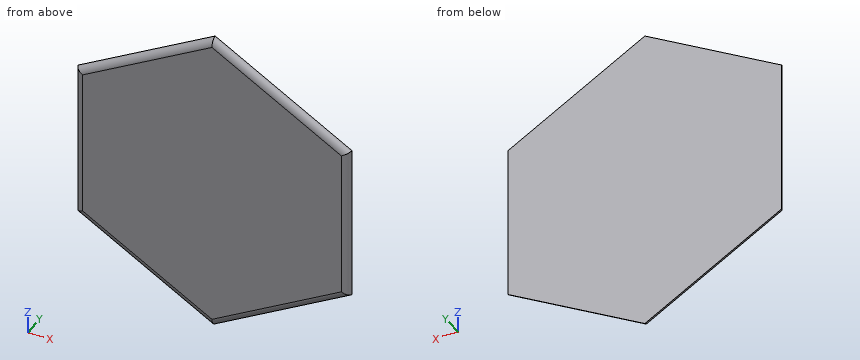
from build123d import *

# Parameters (mm, degrees)
F1_DEPTH     = 4
F2_T1_DEPTH  = 128.417945882
F2_T3_DEPTH  = 128.417945882
F2_T5_DEPTH  = 128.417945882
F2_T7_DEPTH  = 128.417945882
F2_T9_DEPTH  = 128.417945882
F2_T11_DEPTH = 128.417945882


# Not quite as in the source:
# - a fillet or chamfer that OpenCascade refuses, or shapes differently, is made with other operations: its cross-section is extruded or revolved along the edge and cut away or added


with BuildPart() as f1:
    # F0 (on Front) → F1 (new body)
    with BuildSketch(Plane.XZ):
        Polygon((89.9928545723, 51.9738985062), (-0.0142891539, 103.9230474718), (-90.0071437262, 51.9491489656), (-89.9928545723, -51.9738985062), (0.0142891539, -103.9230474718), (90.0071437262, -51.9491489656), align=None)
    extrude(amount=F1_DEPTH)

    # F2: fillet of radius 5 on 6 edges, made by hand

    # F2_s2 → F2_t1 (cut)
    with BuildSketch(Plane(origin=(-0.0088285699, 0, 64.208972334), x_dir=(0, 1, 0), z_dir=(0.0001374974, 0, -0.9999999905))):
        with BuildLine():
            ThreePointArc((0, -90), (-2.8729833462, -88.2632981746), (-4, -85.1010205144))
            Line((-4, -85.1010205144), (-4, -90))
            Line((-4, -90), (0, -90))
        make_face()
    extrude(amount=F2_T1_DEPTH, mode=Mode.SUBTRACT)

    # F2_s4 → F2_t3 (cut)
    with BuildSketch(Plane(origin=(55.6021869072, 0, 32.1121319328), x_dir=(0, 1, 0), z_dir=(-0.8659566469, 0, -0.5001190716))):
        with BuildLine():
            ThreePointArc((0, -90), (-2.8729833462, -88.2632981746), (-4, -85.1010205144))
            Line((-4, -85.1010205144), (-4, -90))
            Line((-4, -90), (0, -90))
        make_face()
    extrude(amount=F2_T3_DEPTH, mode=Mode.SUBTRACT)

    # F2_s6 → F2_t5 (cut)
    with BuildSketch(Plane(origin=(55.6110154771, 0, -32.0968404012), x_dir=(0, 1, 0), z_dir=(-0.8660941443, 0, 0.499880919))):
        with BuildLine():
            ThreePointArc((0, -90), (-2.8729833462, -88.2632981746), (-4, -85.1010205144))
            Line((-4, -85.1010205144), (-4, -90))
            Line((-4, -90), (0, -90))
        make_face()
    extrude(amount=F2_T5_DEPTH, mode=Mode.SUBTRACT)

    # F2_s8 → F2_t7 (cut)
    with BuildSketch(Plane(origin=(0.0088285699, 0, -64.208972334), x_dir=(0, 1, 0), z_dir=(-0.0001374974, 0, 0.9999999905))):
        with BuildLine():
            ThreePointArc((0, -90), (-2.8729833462, -88.2632981746), (-4, -85.1010205144))
            Line((-4, -85.1010205144), (-4, -90))
            Line((-4, -90), (0, -90))
        make_face()
    extrude(amount=F2_T7_DEPTH, mode=Mode.SUBTRACT)

    # F2_s10 → F2_t9 (cut)
    with BuildSketch(Plane(origin=(-55.6021869072, 0, -32.1121319328), x_dir=(0, 1, 0), z_dir=(0.8659566469, 0, 0.5001190716))):
        with BuildLine():
            ThreePointArc((0, -90), (-2.8729833462, -88.2632981746), (-4, -85.1010205144))
            Line((-4, -85.1010205144), (-4, -90))
            Line((-4, -90), (0, -90))
        make_face()
    extrude(amount=F2_T9_DEPTH, mode=Mode.SUBTRACT)

    # F2_s12 → F2_t11 (cut)
    with BuildSketch(Plane(origin=(-55.6110154771, 0, 32.0968404012), x_dir=(0, 1, 0), z_dir=(0.8660941443, 0, -0.499880919))):
        with BuildLine():
            ThreePointArc((0, -90), (-2.8729833462, -88.2632981746), (-4, -85.1010205144))
            Line((-4, -85.1010205144), (-4, -90))
            Line((-4, -90), (0, -90))
        make_face()
    extrude(amount=F2_T11_DEPTH, mode=Mode.SUBTRACT)


solid = f1.part
Source: CAD feature listing. Evaluate the final solid. Frame: model axes, mm. Round coordinates to 2 decimals unless told otherwise and drop trailing zeros. Loops run counter-clockwise (first coordinate to the right, second up) from the corner with the lowest first, then second, coordinate; pieces in that order, holes last. Notation, with made-up numbers: (-16.5, -12.75) -> (7.5, -12.75) arc R15 cw to (7.5, -3.75) -> close; hole circle Ø2 at (73.5, 59). An arc over 180 degrees is marked (long way). Answer as a JSON object with one key per item and string values. Group by question number.
Q1. Ray query, line 1 (Z direction, x = 9, y = -1.25); line 2 (X direction, y = -2.55, z = -21.5); line 3 (Z direction, x = -67.5, y = -0.65). Return the intervals inside material, ascending. Write a range as from..to.
Q2. Contact query for flat-ended pins moving along their axis: P1, Ø1, axis at x = 31.5, y = -2.5, coming from the +Z side; P2, Ø10, axis at x = 68.5, z = 16, coming from the +Y side; P3, Ø1, axis at y = -1, z = -1, coming from the +X side. Output: stop coordinate, or through.
Q3. Section query A-A (y = -1.5). Output: boundary loops of the cut face in (x, z), plus the area to 3 significant figures.
Completed:
{
 "1": {"line 1": "-98.23..98.22", "line 2": "-88.62..88.62", "line 3": "-64.75..64.74"},
 "2": {"P1": "z = 84.78", "P2": "y = 0", "P3": "x = 89.87"},
 "3": {"outline": "(-89.44, 51.62) -> (-89.42, -51.65) -> (0.01, -103.27) -> (89.44, -51.62) -> (89.42, 51.65) -> (-0.01, 103.27) -> close", "area": "27,700 mm²"}
}
